Geometry check sheet. Reference: the model listing, model coordinates, mm. Face numbers are marked on the shaded views. A direction names the side the tool comes from. Round coordinates to 2 decimals unless told otherwise and drop trailing zeros. Order: outer loops, then holes, each group sorted by start corner. A loop starts at its lowest first (then second) coordinate and runs counter-clockwise, first axis right, second up. Notation, with made-up numbers: (40, 12) -> (56, 12) arc R21 cw to (56, 20) -> close; hole circle Ø5 at (82.25, -34). An arc over 180 degrees is marked (long way). Answer as a JSON object with one key per item and string values. Group by question number.
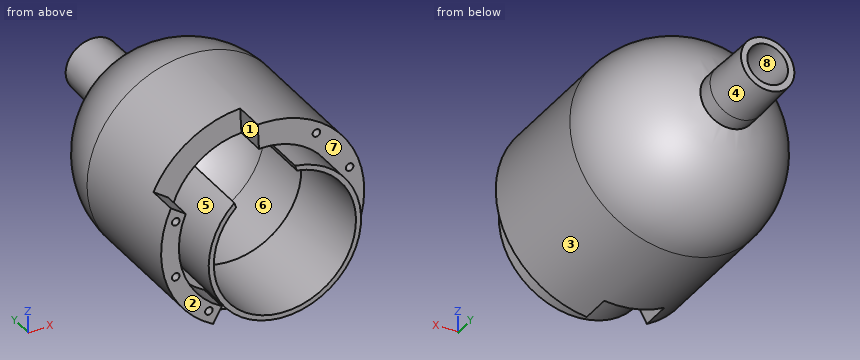
from build123d import *

# Parameters (mm, degrees)
ESBO_O1_R                     = 40
ESBO_O1_R_2                   = 30
RESSALTO_EXTRUS_O1_DEPTH      = 50
ESBO_O2_R                     = 1.5
CORTE_EXTRUS_O1_DEPTH         = 10
CORTE_EXTRUS_O2_DEPTH         = 11.84997677
RESSALTO_EXTRUS_O2_DEPTH      = 26.84997677
RESSALTO_EXTRUS_O2_DEPTH_BACK = 10
REVOLU_O1_ANGLE               = 180
RESSALTO_EXTRUS_O5_DEPTH      = 5
RESSALTO_EXTRUS_O5_DEPTH_BACK = 2
ESBO_O10_R                    = 11
ESBO_O13_R                    = 8
CORTE_EXTRUS_O4_DEPTH         = 40
ESCALA1_SCALE                 = 0.681818182


# Read off the part's stored shape, not the designer's step: Limites1
with BuildPart() as part:
    # Esboço1 → Ressalto-extrusão1 (new body)
    with BuildSketch(Plane(origin=(0, 0, 0), x_dir=(1, 0, 0), z_dir=(0, 1, 0))):
        with Locations(Location((0, 0, 0), (0, 0, 270))):
            Circle(ESBO_O1_R)
        with Locations(Location((0, 0, 0), (0, 0, 270))):
            Circle(ESBO_O1_R_2, mode=Mode.SUBTRACT)
    extrude(amount=RESSALTO_EXTRUS_O1_DEPTH)

    # Esboço2 → Corte-extrusão1 (cut)
    with BuildSketch(Plane(origin=(0, 0, 0), x_dir=(-1, 0, 0), z_dir=(0, -1, 0))):
        with Locations(Location((-21.160269083, -29.124611797, 0), (0, 0, 90))):
            Circle(ESBO_O2_R)
        with Locations(Location((-34.238034587, -11.124611797, 0), (0, 0, 90))):
            Circle(ESBO_O2_R)
        with Locations(Location((-34.238034587, 11.124611797, 0), (0, 0, 90))):
            Circle(ESBO_O2_R)
        with Locations(Location((21.160269083, 29.124611797, 0), (0, 0, 90))):
            Circle(ESBO_O2_R)
        with Locations(Location((34.238034587, 11.124611797, 0), (0, 0, 90))):
            Circle(ESBO_O2_R)
        with Locations(Location((34.238034587, -11.124611797, 0), (0, 0, 90))):
            Circle(ESBO_O2_R)
    extrude(amount=-CORTE_EXTRUS_O1_DEPTH, mode=Mode.SUBTRACT)

    # Esboço3 → Corte-extrusão2 (cut)
    with BuildSketch(Plane(origin=(0, 0, 0), x_dir=(-1, 0, 0), z_dir=(0, -1, 0))):
        with BuildLine():
            ThreePointArc((30.293924668, -13.087327008), (31.253408489, 10.593604572), (16.092357529, 28.81034587))
            Line((16.092357529, 28.81034587), (19.505887914, 34.921631358))
            ThreePointArc((19.505887914, 34.921631358), (8.030354378, 39.185627576), (-4.197370073, 39.779166463))
            Line((-4.197370073, 39.779166463), (-3.148027555, 29.834374847))
            ThreePointArc((-3.148027555, 29.834374847), (29.911212101, 2.306380417), (1.462902849, -29.964310692))
            Line((1.462902849, -29.964310692), (1.950537132, -39.952414256))
            ThreePointArc((1.950537132, -39.952414256), (22.185986252, -33.283359416), (36.126859334, -17.171197823))
            Line((36.126859334, -17.171197823), (30.293924668, -13.087327008))
        make_face()
    extrude(amount=-CORTE_EXTRUS_O2_DEPTH, mode=Mode.SUBTRACT)

    # Esboço4 → Ressalto-extrusão2 (add, two sides: drawn at the far end of the back side and taken through both)
    with BuildSketch(Plane(origin=(0, 11.84997677, 0), x_dir=(-1, 0, 0), z_dir=(0, -1, 0)).offset(-RESSALTO_EXTRUS_O2_DEPTH_BACK)):
        with BuildLine():
            Line((-4.008838629, -29.730947056), (-4.700362463, -27.602655537))
            ThreePointArc((-4.700362463, -27.602655537), (-8.119302432, 26.79695744), (19.230258499, -20.351834268))
            Line((19.230258499, -20.351834268), (19.909240802, -22.441526924))
            ThreePointArc((19.909240802, -22.441526924), (-8.745833796, 28.696870757), (-4.008838629, -29.730947056))
        make_face()
    extrude(amount=RESSALTO_EXTRUS_O2_DEPTH + RESSALTO_EXTRUS_O2_DEPTH_BACK)

    # Esboço9 → Revolução1 (revolve)
    with BuildSketch(Plane(origin=(0, 50, 0), x_dir=(1, 0, 0), z_dir=(0, 1, 0))):
        with BuildLine():
            Line((-40, 0), (-30, 0))
            ThreePointArc((-30, 0), (0, 30), (30, 0))
            Line((30, 0), (40, 0))
            ThreePointArc((40, 0), (0, 40), (-40, 0))
        make_face()
    revolve(axis=Axis((-40, 50, 0), (1, 0, 0)), revolution_arc=REVOLU_O1_ANGLE)

    # Esboço10 → Ressalto-extrusão5 (add, two sides: drawn at the far end of the back side and taken through both)
    with BuildSketch(Plane(origin=(0, 90, 0), x_dir=(1, 0, 0), z_dir=(0, 1, 0)).offset(-RESSALTO_EXTRUS_O5_DEPTH_BACK)):
        with Locations(Location((0, 0, 0), (0, 0, 270))):
            Circle(ESBO_O10_R)
    extrude(amount=RESSALTO_EXTRUS_O5_DEPTH + RESSALTO_EXTRUS_O5_DEPTH_BACK)

    # Limites1 outline → Limites1 (revolve)
    with BuildSketch(Plane.XY):
        Polygon((11, 95), (10.5, 115), (0, 115), (0, 95), align=None)
    revolve(axis=Axis((0, 0, 0), (0, 1, 0)))

    # Esboço13 → Corte-extrusão4 (cut)
    with BuildSketch(Plane(origin=(0, 115, 0), x_dir=(1, 0, 0), z_dir=(0, 1, 0))):
        with Locations(Location((0, 0, 0), (0, 0, 270))):
            Circle(ESBO_O13_R)
    extrude(amount=-CORTE_EXTRUS_O4_DEPTH, mode=Mode.SUBTRACT)


with BuildPart() as part_1:
    # Escala1: scaled about (0, 0, 0)
    add(part.part.scale(ESCALA1_SCALE))


solid = part_1.part
Item 1: Sectioned sample at B-B, the plane x = 0. Enter the section's corners in (y, z).
Item 2: Thickness scan on L1, parallel to Z at x = 0, y = 7; L2, parallel to Z at x = 8, y = 12; L3, parallel to X at y = 37, z = -10.5. Record the ranges inside material, lowest first.
Item 3: Set-up check for the marked faces 4, 5, 6, 7 and 8: record each of +Z, -Z, +X, -X, +Y, -Y from which the full face is reachable in a straight line by a thin tool's end or side.
Item 4: Depth check by flat-ended pin: pin 1 Ø2.5 at (x, z) = (-14.43, -19.86) entering from +Y; pin 2 Ø8 at (y, z) = (27, 13.5) entering from +X; pin 3 Ø1 at (x, z) = (14.5, 20) entering from -Y. Enter the tip coordinate at first touch or a pass-through.
Item 5: Sectioned sample at D-D, the plane z = -13. Enter the section's corners in (x, y), then the cut area to 3 significant figures.
Item 6: Mould release check, pull along Z, two halves, no side actions. Record for the marked faces 1, 2 and 3: pulls with the +Z half, pulls with the -Z half, needs draft (parallel to the pull), parting line crosses it, or undercut.
Item 7: Sectioned sample at C-C, the plane y = 72. Enter the section's corners in (x, z), then the cut area to 3 significant figures.
Item 8: Sectioned sample at A-A, the plane z = 0. Enter the section's corners in (x, y).
Result:
{
 "1": {"outline": "(-10.23, -20.45) -> (8.08, -20.45) -> (8.08, -27.27) -> (34.09, -27.27) arc R27.27 ccw to (60.31, -7.5) -> (64.77, -7.5) -> (78.41, -7.16) -> (78.41, -5.45) -> (53.8, -5.45) arc R20.45 cw to (34.09, -20.45) -> (14.9, -20.45) -> (14.9, -19.09) -> (-10.23, -19.09) -> close; (0, 20.45) -> (34.09, 20.45) arc R20.45 cw to (53.8, 5.45) -> (78.41, 5.45) -> (78.41, 7.16) -> (64.77, 7.5) -> (60.31, 7.5) arc R27.27 ccw to (34.09, 27.27) -> (0, 27.27) -> close"},
 "2": {"L1": "z = -20.45 to -19.09, 20.45 to 27.27", "L2": "z = -26.07 to -17.33, 17.33 to 26.07", "L3": "x = -25 to -17.31, 17.31 to 25"},
 "3": {"face 4": "+Y", "face 5": "-Y", "face 6": "none", "face 7": "+X, -Y", "face 8": "+Y, -Y"},
 "4": {"pin 1": "stops at y = 48.27", "pin 2": "stops at x = 25.56", "pin 3": "stops at y = 6.82"},
 "5": {"outline": "(-23.98, 0) -> (-18.36, 0) -> (-18.36, 8.08) -> (-15.79, 8.08) -> (-15.79, -10.23) -> (-13.98, -10.23) -> (-13.98, 14.9) -> (-15.79, 14.9) -> (-15.79, 34.09) arc R15.79 cw to (15.79, 34.09) -> (15.79, 14.9) -> (13.98, 14.9) -> (13.98, -10.23) -> (15.79, -10.23) -> (15.79, 0) -> (23.98, 0) -> (23.98, 34.09) arc R23.98 ccw to (-23.98, 34.09) -> close", "area": "1,140 mm2"},
 "6": {"face 1": "undercut", "face 2": "needs draft", "face 3": "parting line crosses it"},
 "7": {"outline": "circle Ø14.64 at (0, 0); hole circle Ø10.91 at (0, 0)", "area": "74.8 mm2"},
 "8": {"outline": "(-27.27, 0) -> (-22.5, 0) -> (-22.5, 8.08) -> (-20.45, 8.08) -> (-20.45, -10.23) -> (-19.09, -10.23) -> (-19.09, 14.9) -> (-20.45, 14.9) -> (-20.45, 34.09) arc R20.45 cw to (-5.45, 53.8) -> (-5.45, 78.41) -> (-7.16, 78.41) -> (-7.5, 64.77) -> (-7.5, 60.31) arc R27.27 ccw to (-27.27, 34.09) -> close; (5.45, 53.8) arc R20.45 cw to (20.45, 34.09) -> (20.45, 14.9) -> (19.09, 14.9) -> (19.09, -10.23) -> (20.45, -10.23) -> (20.45, 0) -> (27.27, 0) -> (27.27, 34.09) arc R27.27 ccw to (7.5, 60.31) -> (7.5, 64.77) -> (7.16, 78.41) -> (5.45, 78.41) -> close"}
}
